For this review, take the finished solid that the model builds, in its own axes (mm). Face numbers are marked on the shaded views. Give positions to 0.01 mm unless a question says otherwise; leave off trailing zeros. Write each loop counter-clockwise with the first axis right and the second up, starting at its lowest first coordinate (ties: lowest second). Pieces come first, ordered by that corner, then holes. Notation, with made-up numbers: M 17,29.5 L 26,29.5 A8 cw 26,33.5 Z; hole C 58.5,51.5 d10. An arc over 180 degrees is marked long. One line per item, written item: value. Start each with the question number.
Item 1: Mouldability with a two-part tool opening along Z and no side actions: class the marked faces 1, 2 and 3 as released by +Z, released by -Z, zero draft, split by the parting line, or undercut.
Item 2: Consider section C-C, the plane x = 1.85. Write out the cut boundary in (y, z).
Item 3: Clearance check with flat-ended pins moving along their axes: pin 1 Ø0.7 at (x, y) = (1, 4.5) entering from +Z (3 decimals); pin 2 Ø0.7 at (x, y) = (1.5, 4.5) entering from -Z (3 decimals); pin 3 Ø0.8 at (x, z) = (1, -10) entering from +Y; pin 4 Ø2 at (y, z) = (3.5, -14.5) entering from +X. State where each tip first meets the part, or that it passes through.
Item 4: Consider section A-A, the plane y = 5. Write out the cut boundary in (x, z).
Item 5: To check wall thickness, follow probe 1 along Y at (x, z) = (0.55, -5); probe 2 along X at (y, z) = (4.55, -1); probe 3 along X at (y, z) = (2.65, -8.5). State the ranges of each line that lie inside material, in increasing order.
Item 6: Consider section B-B, the plane y = 3.1. Write out the cut boundary in (x, z) (3 decimals), and give its area (3 significant figures).
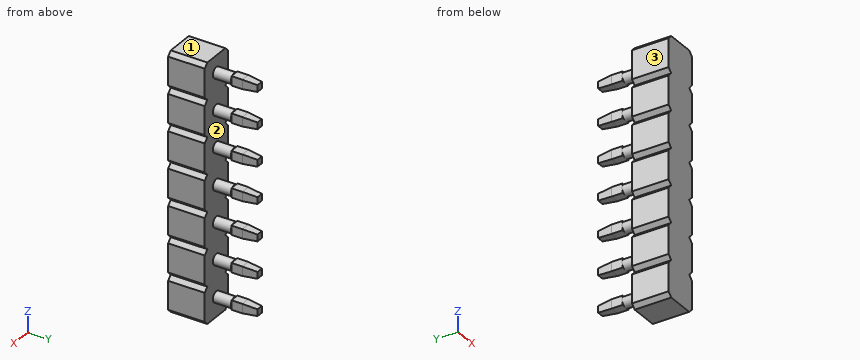
```python
from build123d import *
from OCP.BRepFilletAPI import BRepFilletAPI_MakeChamfer

# Parameters (mm, degrees)
SKETCH1_W           = 2.5
SKETCH1_H           = 2.54
BOSS_EXTRUDE1_DEPTH = 2.54
SKETCH3_R           = 0.375
BOSS_EXTRUDE2_DEPTH = 1.25
SKETCH4_W           = 0.64
SKETCH4_H           = 0.64
BOSS_EXTRUDE3_DEPTH = 1.76
CUT_EXTRUDE1_DEPTH  = 2.54
LPATTERN5_COUNT     = 7
LPATTERN5_PITCH     = 2.54
CHAMFER3_SIZE       = 1
CHAMFER3_SIZE2      = 0.087488664


with BuildPart() as part:
    # Sketch1 → Boss-Extrude1 (new body)
    with BuildSketch(Plane(origin=(0, 0, 0), x_dir=(1, 0, 0), z_dir=(0, 1, 0))):
        with Locations((1.25, 1.27)):
            Rectangle(SKETCH1_W, SKETCH1_H)
    boss_extrude1 = extrude(amount=BOSS_EXTRUDE1_DEPTH)

    # Sketch3 → Boss-Extrude2 (add)
    with BuildSketch(Plane(origin=(0, 2.54, 0), x_dir=(1, 0, 0), z_dir=(0, 1, 0))):
        with Locations(Location((1.25, 1.165, 0), (0, 0, 270))):
            Circle(SKETCH3_R)
    boss_extrude2 = extrude(amount=BOSS_EXTRUDE2_DEPTH)

    # Sketch4 → Boss-Extrude3 (add)
    with BuildSketch(Plane(origin=(0, 3.79, 0), x_dir=(1, 0, 0), z_dir=(0, 1, 0))):
        with Locations((1.25, 1.165)):
            Rectangle(SKETCH4_W, SKETCH4_H)
    boss_extrude3 = extrude(amount=BOSS_EXTRUDE3_DEPTH)

    # Sketch5 → Cut-Extrude1 (cut)
    with BuildSketch(Plane(origin=(0, 2.54, 0), x_dir=(1, 0, 0), z_dir=(0, 1, 0))):
        Polygon((0.282842712, 2.54), (0, 2.257157288), (0, 2.54), align=None)
        Polygon((2.5, 2.54), (2.5, 2.257157288), (2.217157288, 2.54), align=None)
        Polygon((2.5, 0), (2.5, 0.282842712), (2.217157288, 0), align=None)
        Polygon((0, 0), (0, 0.282842712), (0.282842712, 0), align=None)
    cut_extrude1 = extrude(amount=-CUT_EXTRUDE1_DEPTH, mode=Mode.SUBTRACT)

    # LPattern5: Boss-Extrude1, Boss-Extrude2, Boss-Extrude3, Cut-Extrude1 ×7
    with Locations(*[(0, 0, -i * LPATTERN5_PITCH) for i in range(1, LPATTERN5_COUNT)]):
        add(boss_extrude1)
        add(boss_extrude2)
        add(boss_extrude3)
        add(cut_extrude1, mode=Mode.SUBTRACT)

    # Chamfer3: one chamfer whose edges measure the first distance from different faces: ONE call of the kernel's chamfer builder (chamfer() names one face for all edges)
    chamfer3_edges_1 = [part.edges().sort_by_distance(p)[0] for p in [
        (1.57, 5.55, -3.705),
    ]]
    chamfer3_side_1 = [part.faces().sort_by_distance(p)[0] for p in [
        (1.57, 4.67, -3.705),
    ]]
    chamfer3_edges_2 = [part.edges().sort_by_distance(p)[0] for p in [
        (1.25, 5.55, -4.025),
    ]]
    chamfer3_side_2 = [part.faces().sort_by_distance(p)[0] for p in [
        (1.25, 4.67, -4.025),
    ]]
    chamfer3_edges_3 = [part.edges().sort_by_distance(p)[0] for p in [
        (0.93, 5.55, -3.705),
    ]]
    chamfer3_side_3 = [part.faces().sort_by_distance(p)[0] for p in [
        (0.93, 4.67, -3.705),
    ]]
    chamfer3_edges_4 = [part.edges().sort_by_distance(p)[0] for p in [
        (1.25, 5.55, -3.385),
    ]]
    chamfer3_side_4 = [part.faces().sort_by_distance(p)[0] for p in [
        (1.25, 4.67, -3.385),
    ]]
    chamfer3_edges_5 = [part.edges().sort_by_distance(p)[0] for p in [
        (1.57, 5.55, -6.245),
    ]]
    chamfer3_side_5 = [part.faces().sort_by_distance(p)[0] for p in [
        (1.57, 4.67, -6.245),
    ]]
    chamfer3_edges_6 = [part.edges().sort_by_distance(p)[0] for p in [
        (1.25, 5.55, -6.565),
    ]]
    chamfer3_side_6 = [part.faces().sort_by_distance(p)[0] for p in [
        (1.25, 4.67, -6.565),
    ]]
    chamfer3_edges_7 = [part.edges().sort_by_distance(p)[0] for p in [
        (0.93, 5.55, -6.245),
    ]]
    chamfer3_side_7 = [part.faces().sort_by_distance(p)[0] for p in [
        (0.93, 4.67, -6.245),
    ]]
    chamfer3_edges_8 = [part.edges().sort_by_distance(p)[0] for p in [
        (1.25, 5.55, -5.925),
    ]]
    chamfer3_side_8 = [part.faces().sort_by_distance(p)[0] for p in [
        (1.25, 4.67, -5.925),
    ]]
    chamfer3_edges_9 = [part.edges().sort_by_distance(p)[0] for p in [
        (1.57, 5.55, -8.785),
    ]]
    chamfer3_side_9 = [part.faces().sort_by_distance(p)[0] for p in [
        (1.57, 4.67, -8.785),
    ]]
    chamfer3_edges_10 = [part.edges().sort_by_distance(p)[0] for p in [
        (1.25, 5.55, -9.105),
    ]]
    chamfer3_side_10 = [part.faces().sort_by_distance(p)[0] for p in [
        (1.25, 4.67, -9.105),
    ]]
    chamfer3_edges_11 = [part.edges().sort_by_distance(p)[0] for p in [
        (0.93, 5.55, -8.785),
    ]]
    chamfer3_side_11 = [part.faces().sort_by_distance(p)[0] for p in [
        (0.93, 4.67, -8.785),
    ]]
    chamfer3_edges_12 = [part.edges().sort_by_distance(p)[0] for p in [
        (1.25, 5.55, -8.465),
    ]]
    chamfer3_side_12 = [part.faces().sort_by_distance(p)[0] for p in [
        (1.25, 4.67, -8.465),
    ]]
    chamfer3_edges_13 = [part.edges().sort_by_distance(p)[0] for p in [
        (1.57, 5.55, -11.325),
    ]]
    chamfer3_side_13 = [part.faces().sort_by_distance(p)[0] for p in [
        (1.57, 4.67, -11.325),
    ]]
    chamfer3_edges_14 = [part.edges().sort_by_distance(p)[0] for p in [
        (1.25, 5.55, -11.645),
    ]]
    chamfer3_side_14 = [part.faces().sort_by_distance(p)[0] for p in [
        (1.25, 4.67, -11.645),
    ]]
    chamfer3_edges_15 = [part.edges().sort_by_distance(p)[0] for p in [
        (0.93, 5.55, -11.325),
    ]]
    chamfer3_side_15 = [part.faces().sort_by_distance(p)[0] for p in [
        (0.93, 4.67, -11.325),
    ]]
    chamfer3_edges_16 = [part.edges().sort_by_distance(p)[0] for p in [
        (1.25, 5.55, -11.005),
    ]]
    chamfer3_side_16 = [part.faces().sort_by_distance(p)[0] for p in [
        (1.25, 4.67, -11.005),
    ]]
    chamfer3_edges_17 = [part.edges().sort_by_distance(p)[0] for p in [
        (1.57, 5.55, -13.865),
    ]]
    chamfer3_side_17 = [part.faces().sort_by_distance(p)[0] for p in [
        (1.57, 4.67, -13.865),
    ]]
    chamfer3_edges_18 = [part.edges().sort_by_distance(p)[0] for p in [
        (1.25, 5.55, -14.185),
    ]]
    chamfer3_side_18 = [part.faces().sort_by_distance(p)[0] for p in [
        (1.25, 4.67, -14.185),
    ]]
    chamfer3_edges_19 = [part.edges().sort_by_distance(p)[0] for p in [
        (0.93, 5.55, -13.865),
    ]]
    chamfer3_side_19 = [part.faces().sort_by_distance(p)[0] for p in [
        (0.93, 4.67, -13.865),
    ]]
    chamfer3_edges_20 = [part.edges().sort_by_distance(p)[0] for p in [
        (1.25, 5.55, -13.545),
    ]]
    chamfer3_side_20 = [part.faces().sort_by_distance(p)[0] for p in [
        (1.25, 4.67, -13.545),
    ]]
    chamfer3_edges_21 = [part.edges().sort_by_distance(p)[0] for p in [
        (1.57, 5.55, -16.405),
    ]]
    chamfer3_side_21 = [part.faces().sort_by_distance(p)[0] for p in [
        (1.57, 4.67, -16.405),
    ]]
    chamfer3_edges_22 = [part.edges().sort_by_distance(p)[0] for p in [
        (1.25, 5.55, -16.725),
    ]]
    chamfer3_side_22 = [part.faces().sort_by_distance(p)[0] for p in [
        (1.25, 4.67, -16.725),
    ]]
    chamfer3_edges_23 = [part.edges().sort_by_distance(p)[0] for p in [
        (0.93, 5.55, -16.405),
    ]]
    chamfer3_side_23 = [part.faces().sort_by_distance(p)[0] for p in [
        (0.93, 4.67, -16.405),
    ]]
    chamfer3_edges_24 = [part.edges().sort_by_distance(p)[0] for p in [
        (1.25, 5.55, -16.085),
    ]]
    chamfer3_side_24 = [part.faces().sort_by_distance(p)[0] for p in [
        (1.25, 4.67, -16.085),
    ]]
    chamfer3_edges_25 = [part.edges().sort_by_distance(p)[0] for p in [
        (1.57, 5.55, -1.165),
    ]]
    chamfer3_side_25 = [part.faces().sort_by_distance(p)[0] for p in [
        (1.57, 4.67, -1.165),
    ]]
    chamfer3_edges_26 = [part.edges().sort_by_distance(p)[0] for p in [
        (1.25, 5.55, -1.485),
    ]]
    chamfer3_side_26 = [part.faces().sort_by_distance(p)[0] for p in [
        (1.25, 4.67, -1.485),
    ]]
    chamfer3_edges_27 = [part.edges().sort_by_distance(p)[0] for p in [
        (0.93, 5.55, -1.165),
    ]]
    chamfer3_side_27 = [part.faces().sort_by_distance(p)[0] for p in [
        (0.93, 4.67, -1.165),
    ]]
    chamfer3_edges_28 = [part.edges().sort_by_distance(p)[0] for p in [
        (1.25, 5.55, -0.845),
    ]]
    chamfer3_side_28 = [part.faces().sort_by_distance(p)[0] for p in [
        (1.25, 4.67, -0.845),
    ]]
    chamfer3 = BRepFilletAPI_MakeChamfer(part.part.solid().wrapped)
    for e in chamfer3_edges_1:
        chamfer3.Add(CHAMFER3_SIZE, CHAMFER3_SIZE2, e.wrapped, chamfer3_side_1[0].wrapped)  # the first distance lies on this face
    for e in chamfer3_edges_2:
        chamfer3.Add(CHAMFER3_SIZE, CHAMFER3_SIZE2, e.wrapped, chamfer3_side_2[0].wrapped)  # the first distance lies on this face
    for e in chamfer3_edges_3:
        chamfer3.Add(CHAMFER3_SIZE, CHAMFER3_SIZE2, e.wrapped, chamfer3_side_3[0].wrapped)  # the first distance lies on this face
    for e in chamfer3_edges_4:
        chamfer3.Add(CHAMFER3_SIZE, CHAMFER3_SIZE2, e.wrapped, chamfer3_side_4[0].wrapped)  # the first distance lies on this face
    for e in chamfer3_edges_5:
        chamfer3.Add(CHAMFER3_SIZE, CHAMFER3_SIZE2, e.wrapped, chamfer3_side_5[0].wrapped)  # the first distance lies on this face
    for e in chamfer3_edges_6:
        chamfer3.Add(CHAMFER3_SIZE, CHAMFER3_SIZE2, e.wrapped, chamfer3_side_6[0].wrapped)  # the first distance lies on this face
    for e in chamfer3_edges_7:
        chamfer3.Add(CHAMFER3_SIZE, CHAMFER3_SIZE2, e.wrapped, chamfer3_side_7[0].wrapped)  # the first distance lies on this face
    for e in chamfer3_edges_8:
        chamfer3.Add(CHAMFER3_SIZE, CHAMFER3_SIZE2, e.wrapped, chamfer3_side_8[0].wrapped)  # the first distance lies on this face
    for e in chamfer3_edges_9:
        chamfer3.Add(CHAMFER3_SIZE, CHAMFER3_SIZE2, e.wrapped, chamfer3_side_9[0].wrapped)  # the first distance lies on this face
    for e in chamfer3_edges_10:
        chamfer3.Add(CHAMFER3_SIZE, CHAMFER3_SIZE2, e.wrapped, chamfer3_side_10[0].wrapped)  # the first distance lies on this face
    for e in chamfer3_edges_11:
        chamfer3.Add(CHAMFER3_SIZE, CHAMFER3_SIZE2, e.wrapped, chamfer3_side_11[0].wrapped)  # the first distance lies on this face
    for e in chamfer3_edges_12:
        chamfer3.Add(CHAMFER3_SIZE, CHAMFER3_SIZE2, e.wrapped, chamfer3_side_12[0].wrapped)  # the first distance lies on this face
    for e in chamfer3_edges_13:
        chamfer3.Add(CHAMFER3_SIZE, CHAMFER3_SIZE2, e.wrapped, chamfer3_side_13[0].wrapped)  # the first distance lies on this face
    for e in chamfer3_edges_14:
        chamfer3.Add(CHAMFER3_SIZE, CHAMFER3_SIZE2, e.wrapped, chamfer3_side_14[0].wrapped)  # the first distance lies on this face
    for e in chamfer3_edges_15:
        chamfer3.Add(CHAMFER3_SIZE, CHAMFER3_SIZE2, e.wrapped, chamfer3_side_15[0].wrapped)  # the first distance lies on this face
    for e in chamfer3_edges_16:
        chamfer3.Add(CHAMFER3_SIZE, CHAMFER3_SIZE2, e.wrapped, chamfer3_side_16[0].wrapped)  # the first distance lies on this face
    for e in chamfer3_edges_17:
        chamfer3.Add(CHAMFER3_SIZE, CHAMFER3_SIZE2, e.wrapped, chamfer3_side_17[0].wrapped)  # the first distance lies on this face
    for e in chamfer3_edges_18:
        chamfer3.Add(CHAMFER3_SIZE, CHAMFER3_SIZE2, e.wrapped, chamfer3_side_18[0].wrapped)  # the first distance lies on this face
    for e in chamfer3_edges_19:
        chamfer3.Add(CHAMFER3_SIZE, CHAMFER3_SIZE2, e.wrapped, chamfer3_side_19[0].wrapped)  # the first distance lies on this face
    for e in chamfer3_edges_20:
        chamfer3.Add(CHAMFER3_SIZE, CHAMFER3_SIZE2, e.wrapped, chamfer3_side_20[0].wrapped)  # the first distance lies on this face
    for e in chamfer3_edges_21:
        chamfer3.Add(CHAMFER3_SIZE, CHAMFER3_SIZE2, e.wrapped, chamfer3_side_21[0].wrapped)  # the first distance lies on this face
    for e in chamfer3_edges_22:
        chamfer3.Add(CHAMFER3_SIZE, CHAMFER3_SIZE2, e.wrapped, chamfer3_side_22[0].wrapped)  # the first distance lies on this face
    for e in chamfer3_edges_23:
        chamfer3.Add(CHAMFER3_SIZE, CHAMFER3_SIZE2, e.wrapped, chamfer3_side_23[0].wrapped)  # the first distance lies on this face
    for e in chamfer3_edges_24:
        chamfer3.Add(CHAMFER3_SIZE, CHAMFER3_SIZE2, e.wrapped, chamfer3_side_24[0].wrapped)  # the first distance lies on this face
    for e in chamfer3_edges_25:
        chamfer3.Add(CHAMFER3_SIZE, CHAMFER3_SIZE2, e.wrapped, chamfer3_side_25[0].wrapped)  # the first distance lies on this face
    for e in chamfer3_edges_26:
        chamfer3.Add(CHAMFER3_SIZE, CHAMFER3_SIZE2, e.wrapped, chamfer3_side_26[0].wrapped)  # the first distance lies on this face
    for e in chamfer3_edges_27:
        chamfer3.Add(CHAMFER3_SIZE, CHAMFER3_SIZE2, e.wrapped, chamfer3_side_27[0].wrapped)  # the first distance lies on this face
    for e in chamfer3_edges_28:
        chamfer3.Add(CHAMFER3_SIZE, CHAMFER3_SIZE2, e.wrapped, chamfer3_side_28[0].wrapped)  # the first distance lies on this face
    add(Compound.cast(chamfer3.Shape()), mode=Mode.REPLACE)


solid = part.part
```
Model answer:
1. face 1: released by +Z
1. face 2: undercut
1. face 3: zero draft
2. outline: M 0,-17.78 L 2.54,-17.78 L 2.54,0 L 0,0 Z
3. pin 1: stops at z = -0.845
3. pin 2: stops at z = -16.725
3. pin 3: stops at y = 2.54
3. pin 4: stops at x = 2.5
4. outline: M 0.97,-16.69 L 1.53,-16.69 L 1.53,-16.12 L 0.97,-16.12 Z; M 0.97,-14.15 L 1.53,-14.15 L 1.53,-13.58 L 0.97,-13.58 Z; M 0.97,-11.61 L 1.53,-11.61 L 1.53,-11.04 L 0.97,-11.04 Z; M 0.97,-9.07 L 1.53,-9.07 L 1.53,-8.5 L 0.97,-8.5 Z; M 0.97,-6.53 L 1.53,-6.53 L 1.53,-5.96 L 0.97,-5.96 Z; M 0.97,-3.99 L 1.53,-3.99 L 1.53,-3.42 L 0.97,-3.42 Z; M 0.97,-1.45 L 1.53,-1.45 L 1.53,-0.88 L 0.97,-0.88 Z
5. probe 1: y = 0 to 2.54
5. probe 2: x = 0.93 to 1.57
5. probe 3: x = 1.01 to 1.49
6. outline: C 1.25,-16.405 d0.75; C 1.25,-13.865 d0.75; C 1.25,-11.325 d0.75; C 1.25,-8.785 d0.75; C 1.25,-6.245 d0.75; C 1.25,-3.705 d0.75; C 1.25,-1.165 d0.75
6. area: 3.09 mm2
